from build123d import *

# Parameters (mm, degrees)
SKETCH_1_W          = 27
SKETCH_1_H          = 20.5
EXTRUDE_1_DEPTH     = 15
SKETCH_2_W          = 0.8
SKETCH_2_H          = 4.8
EXTRUDE_2_DEPTH     = 9
CHAMFER_1_SIZE      = 1
SKETCH_3_W          = 31
SKETCH_3_H          = 24
EXTRUDE_3_DEPTH     = 3
CUT_EXTRUDE_1_DEPTH = 17
SKETCH_5_W          = 2
SKETCH_5_H          = 4
EXTRUDE_4_DEPTH     = 15
CHAMFER_2_SIZE      = 0.8
FILLET_1_R          = 2


with BuildPart() as part:
    # Эскиз1 → Бобышка-Вытянуть1 (new body)
    with BuildSketch(Plane(origin=(0, 0, 0), x_dir=(1, 0, 0), z_dir=(0, 1, 0))):
        Rectangle(SKETCH_1_W, SKETCH_1_H)
    extrude(amount=EXTRUDE_1_DEPTH)

    # Эскиз2 → Бобышка-Вытянуть2 (add)
    with BuildSketch(Plane.XZ):
        with Locations((0, 3)):
            Rectangle(SKETCH_2_W, SKETCH_2_H)
        with Locations((-7, -3)):
            Rectangle(SKETCH_2_W, SKETCH_2_H)
        with Locations((7, -3)):
            Rectangle(SKETCH_2_W, SKETCH_2_H)
    extrude(amount=EXTRUDE_2_DEPTH)

    # Фаска1
    chamfer_1_edges = [part.edges().sort_by_distance(p)[0] for p in [
        (-7, -9, -0.6),
        (-7, -9, -5.4),
        (0, -9, 5.4),
        (0, -9, 0.6),
        (7, -9, -0.6),
        (7, -9, -5.4),
    ]]
    chamfer(chamfer_1_edges, length=CHAMFER_1_SIZE)

    # Эскиз3 → Бобышка-Вытянуть3 (add)
    with BuildSketch(Plane(origin=(0, 15, 0), x_dir=(1, 0, 0), z_dir=(0, 1, 0))):
        Rectangle(SKETCH_3_W, SKETCH_3_H)
    extrude(amount=EXTRUDE_3_DEPTH)

    # Эскиз4 → Вырез-Вытянуть1 (cut)
    with BuildSketch(Plane(origin=(0, 18, 0), x_dir=(1, 0, 0), z_dir=(0, 1, 0))):
        Polygon((12, -3), (7, -8), (-7, -8), (-12, -3), (-12, 8), (12, 8), align=None)
    extrude(amount=-CUT_EXTRUDE_1_DEPTH, mode=Mode.SUBTRACT)

    # Эскиз5 → Бобышка-Вытянуть4 (add)
    with BuildSketch(Plane(origin=(0, 1, 0), x_dir=(1, 0, 0), z_dir=(0, 1, 0))):
        with Locations((7, 2)):
            Rectangle(SKETCH_5_W, SKETCH_5_H)
        with Locations((0, -2)):
            Rectangle(SKETCH_5_W, SKETCH_5_H)
        with Locations((-7, 2)):
            Rectangle(SKETCH_5_W, SKETCH_5_H)
    extrude(amount=EXTRUDE_4_DEPTH)

    # Фаска2
    chamfer_2_edges = [part.edges().sort_by_distance(p)[0] for p in [
        (-1, 16, 2),
        (0, 16, 4),
        (1, 16, 2),
        (0, 16, 0),
        (6, 16, -2),
        (7, 16, 0),
        (8, 16, -2),
        (7, 16, -4),
        (-7, 16, -4),
        (-8, 16, -2),
        (-7, 16, 0),
        (-6, 16, -2),
    ]]
    chamfer(chamfer_2_edges, length=CHAMFER_2_SIZE)

    # Скругление1
    fillet_1_edges = [part.edges().sort_by_distance(p)[0] for p in [
        (-15.5, 16.5, -12),
        (-15.5, 16.5, 12),
        (15.5, 16.5, 12),
        (15.5, 16.5, -12),
    ]]
    fillet(fillet_1_edges, radius=FILLET_1_R)


solid = part.part
CAD build for the part. Positions are in the model's coordinates, mm. A direction names the side the tool comes from. Round coordinates to 2 decimals unless told otherwise and drop trailing zeros. Write each loop counter-clockwise with the first axis right and the second up, starting at its lowest first coordinate (ties: lowest second). Pieces come first, ordered by that corner, then holes. Notation, with made-up numbers: (-7, -11) -> (-2, -11) arc R22 ccw to (-2, 0) -> close; hole circle Ø3 at (83, 57). An arc over 180 degrees is marked (long way). Answer as a JSON object with one key per item and string values.
(1) Band-saw the part on B-B, the plane y = -4.25. List the corners of the cut face in (x, z).
Reported:
{"outline": "(-7.4, -5.4) -> (-6.6, -5.4) -> (-6.6, -0.6) -> (-7.4, -0.6) -> close; (-0.4, 0.6) -> (0.4, 0.6) -> (0.4, 5.4) -> (-0.4, 5.4) -> close; (6.6, -5.4) -> (7.4, -5.4) -> (7.4, -0.6) -> (6.6, -0.6) -> close"}
(2) Probe probe 1 along X at (y, z) = (8, 2.25); probe 2 along X at (y, z) = (-5.75, -5); probe 3 along Z at (x, y) = (6.5, 6.25). List the from-to ranges inside material, lowest first. Write a range as [from, to].
Reported:
{"probe 1": "x = [-13.5, -12], [-1, 1], [12, 13.5]", "probe 2": "x = [-7.4, -6.6], [6.6, 7.4]", "probe 3": "z = [-10.25, -8], [-4, 0], [8, 10.25]"}
(3) Which spindle directions (+Z, -Z, +X, -X, +Y, -Y) get a long thin tool onto all of the face, cutting with end or side? Do faces 1 (the face through (-13.5, 7, 0)), 2 (the face through (8, 8, -2)), 3 (the face through (7, -4, -0.6)), 4 (the face through (0, -8.5, 1.1)). Say none if no direction does.
Reported:
{"face 1": "+Z, -Z, -X, -Y", "face 2": "+Y", "face 3": "+Z, +X, -X, -Y", "face 4": "-Z, +X, -X, -Y"}
(4) Band-saw the part on C-C, the plane x = 10. List the corners of the cut face in (y, z).
Reported:
{"outline": "(0, -10.25) -> (15, -10.25) -> (15, -12) -> (18, -12) -> (18, -8) -> (1, -8) -> (1, 5) -> (18, 5) -> (18, 12) -> (15, 12) -> (15, 10.25) -> (0, 10.25) -> close"}
(5) Band-saw the part on A-A, the plane y = 3.75. List the corners of the cut face in (x, z), then the cut area to 4 significant figures.
Reported:
{"outline": "(-13.5, -10.25) -> (13.5, -10.25) -> (13.5, 10.25) -> (-13.5, 10.25) -> close; (-8, -4) -> (-6, -4) -> (-6, 0) -> (-8, 0) -> close; (-1, 0) -> (1, 0) -> (1, 4) -> (-1, 4) -> close; (6, -4) -> (8, -4) -> (8, 0) -> (6, 0) -> close; hole (-12, -8) -> (12, -8) -> (12, 3) -> (7, 8) -> (-7, 8) -> (-12, 3) -> close", "area": "218.5 mm^2"}
(6) Pin check, flat tips, straight feed: P1, Ø3, axis at x = -5, z = -5.5, coming from the +Y side; P2, Ø0.6, axis at x = 0, y = 9, coming from the -Z side; P3, Ø3, axis at y = -2, z = -4.5, coming from the -X side. Stop position of each tip, or through.
Reported:
{"P1": "stops at y = 1", "P2": "stops at z = -10.25", "P3": "stops at x = -7.4"}
(7) Band-saw the part on D-D, the plane x = 4. List the corners of the cut face in (y, z), then the cut area to 4 significant figures.
Reported:
{"outline": "(0, -10.25) -> (15, -10.25) -> (15, -12) -> (18, -12) -> (18, -8) -> (1, -8) -> (1, 8) -> (18, 8) -> (18, 12) -> (15, 12) -> (15, 10.25) -> (0, 10.25) -> close", "area": "107.5 mm^2"}
(8) Two-plate mould, pull along Z, no slides. Class faces 5 (the face through (7, 8, 0)), 6 (the face through (-7.4, -4, -3)), 7 (the face through (0, -8.5, 4.9)): +Z half, -Z half, draft (parallel to the pull), parting line (faces both ways), or undercut.
Reported:
{"face 5": "undercut", "face 6": "draft", "face 7": "+Z half"}
